Autodesk Fusion 360 part; units mm, degrees
sketch "Sketch1" plane through (0, 0, 0) normal (0, 1, 0) x (1, 0, 0)
  line L0 (10, -15) -> (-10, -15)
  line L1 (-10, -15) -> (-10, 6)
  line L2 (-10, 6) -> (10, 6)
  line L3 (10, 6) -> (10, -15)
  dimension "d1" = 21
  dimension "d2" = 20
extrude "Extrude1" add sketch "Sketch1" along normal blind 2
sketch "Sketch2" plane through (0, 2, 0) normal (0, 1, 0) x (-1, 0, 0)
  line L0 (-10, -6) -> (10, -6)
  line L1 (10, -6) -> (10, 15)
  line L2 (10, 15) -> (-10, 15)
  line L3 (-10, 15) -> (-10, -6)
  line L4 (-1, 15) -> (1, 15)
  line L5 (1, 15) -> (1, -6)
  line L6 (1, -6) -> (-1, -6)
  line L7 (-1, -6) -> (-1, 15)
  dimension "d5" = 2
  dimension "d6" = 9
extrude "Extrude2" add sketch "Sketch2" along normal blind 70 contours L0 L2 L4 L5 L6 L7
sketch "Sketch3" plane through (0, 2, 0) normal (0, 1, 0) x (-1, 0, 0)
  line L0 (-1, -6) -> (-1, 15)
  line L1 (-1, 15) -> (-10, 15)
  line L2 (-10, 15) -> (-10, -6)
  line L3 (-10, -6) -> (-1, -6)
  circle A0 centre (-5, 4.5) radius 1.2
  circle A1 centre (5, 4.5) radius 1.2
  line L4 (10, 15) -> (1, 15)
  dimension "d9" = 2.4
  dimension "d10" = 2.4
  dimension "d11" = 10.5
  dimension "d12" = 10.5
  dimension "d19" = 10
extrude "Extrude3" cut sketch "Sketch3" against normal blind 2 contours A0 | A1
fillet "Fillet1" radius 1 6 edges at (10, 2, 4.5) (5.5, 2, 15) (-5.5, 2, 15) (-10, 2, 4.5) (-5.5, 2, -6) (5.5, 2, -6)
fillet "Fillet2" radius 4 2 edges at (0, 72, 15) (0, 72, -6)
Read the model definition and answer for the solid it produces. Units are mm, in the model's axes. A direction names the side the tool comes from. Coordinates: 2 decimals unless noted, no trailing zeros. Loops run counter-clockwise (first coordinate to the right, second up) from the corner with the lowest first, then second, coordinate; pieces in that order, holes last. Notation, with made-up numbers: (13.5, 50.25) - (41.5, 50.25) arc R20 ccw to (41.5, 60.25) - close; hole circle Ø6 at (45, 7.5). An arc over 180 degrees is marked (long way). Answer in a Markdown table with one row per item.
Q1. Find section D-D on x = 5.25. Write down the section's boundary in (y, z), plus the area to 3 significant figures.
Here are the results:
| item | result |
|---|---|
| outline | (0, -6) - (1, -6) arc R1 ccw to (2, -5) - (2, 3.33) - (0, 3.33) - close; (0, 5.67) - (2, 5.67) - (2, 14) arc R1 ccw to (1, 15) - (0, 15) - close |
| area | 36.9 mm^2 |
Q2. Given P1, Ø4, axis at x = 4, z = 6.5, coming from the +Y side; P2, Ø10, axis at y = 32, z = 8, coming from the -X side; P3, Ø5, axis at y = 63, z = 9.5, coming from the +X side; P4, Ø1.4, axis at x = -5, z = 4.5, coming from the -Y side, each flat-ended and moving along its own axis, determine where each tip first touches the part or whether it passes through.
Here are the results:
| item | result |
|---|---|
| P1 | stops at y = 2 |
| P2 | stops at x = -1 |
| P3 | stops at x = 1 |
| P4 | passes through |
Q3. Find section B-B on x = -5. Write down the section's boundary in (y, z).
Here are the results:
| item | result |
|---|---|
| outline | (0, -6) - (1, -6) arc R1 ccw to (2, -5) - (2, 3.3) - (0, 3.3) - close; (0, 5.7) - (2, 5.7) - (2, 14) arc R1 ccw to (1, 15) - (0, 15) - close |
Q4. Straight lines are drawn through the part: line 1 along Z through (x, y) = (-5, 0.7); line 2 along Y through (x, z) = (-6.25, 0); line 3 along X through (y, z) = (57, 4). For each, find the intervals that lie inside material, in ascending order. Write a range as [from, to].
Here are the results:
| item | result |
|---|---|
| line 1 | z = [-6, 3.3], [5.7, 15] |
| line 2 | y = [0, 2] |
| line 3 | x = [-1, 1] |
Q5. Find section C-C on y = 58. Write down the section's boundary in (x, z).
Here are the results:
| item | result |
|---|---|
| outline | (-1, -6) - (1, -6) - (1, 15) - (-1, 15) - close |
Q6. For faces 1 (the flat face through (0, 0, 4)), 2 (the flat face through (7, 2, 4)), 3 (the flat face through (-7, 2, 4)), determine the directions among +Z, -Z, +X, -X, +Y, -Y from which every point of the face is accessible in a straight line to the end or side of a thin tool.
Here are the results:
| item | result |
|---|---|
| face 1 | +Z, -Z, +X, -X, -Y |
| face 2 | +Z, -Z, +X, +Y |
| face 3 | +Z, -Z, -X, +Y |
Q7. The mould has two halves that part along X. Classify faces 4 (the flat face through (1, 36, 4)), 5 (the cylindrical face through (0.014, 70.859, 13.797)), 6 (the cylindrical face through (6.2, 1.01, 4.55)), 7 (the flat face through (-1, 36, 5)): pulls with the +X half, pulls with the -X half, needs draft (parallel to the pull), parting line crosses it, or undercut.
Here are the results:
| item | result |
|---|---|
| face 4 | pulls with the +X half |
| face 5 | needs draft |
| face 6 | undercut |
| face 7 | pulls with the -X half |
Q8. Find section A-A on z = 4.5. Write down the section's boundary in (x, y).
Here are the results:
| item | result |
|---|---|
| outline | (-10, 0) - (-6.2, 0) - (-6.2, 2) - (-9, 2) arc R1 ccw to (-10, 1) - close; (-3.8, 0) - (3.8, 0) - (3.8, 2) - (1, 2) - (1, 72) - (-1, 72) - (-1, 2) - (-3.8, 2) - close; (6.2, 0) - (10, 0) - (10, 1) arc R1 ccw to (9, 2) - (6.2, 2) - close |
